```python
from build123d import *

# Parameters (mm, degrees)
SKETCH1_W                                     = 457.2
SKETCH1_H                                     = 50.8
BOSS_EXTRUDE1_DEPTH                           = 4.7625
SKETCH2_R                                     = 3.175
CUT_EXTRUDE1_DEPTH                            = 244.602
SKETCH3_R                                     = 3.175
CUT_EXTRUDE2_DEPTH                            = 244.602
SKETCH4_R                                     = 3.175
CUT_EXTRUDE3_DEPTH                            = 25.4
CSK_FOR_8_FLAT_HEAD_MACHINE_SCREW1_AT_2_COUNT = 2
CSK_FOR_8_FLAT_HEAD_MACHINE_SCREW1_AT_2_PITCH = 31.75
CSK_FOR_8_FLAT_HEAD_MACHINE_SCREW1_AT_3_COUNT = 2
CSK_FOR_8_FLAT_HEAD_MACHINE_SCREW1_AT_3_PITCH = 68.170141008
CSK_FOR_8_FLAT_HEAD_MACHINE_SCREW1_AT_4_COUNT = 2
CSK_FOR_8_FLAT_HEAD_MACHINE_SCREW1_AT_4_PITCH = 60.325
CSK_FOR_8_FLAT_HEAD_MACHINE_SCREW1_AT_5_COUNT = 2
CSK_FOR_8_FLAT_HEAD_MACHINE_SCREW1_AT_5_PITCH = 304.8
CSK_FOR_8_FLAT_HEAD_MACHINE_SCREW1_AT_6_COUNT = 2
CSK_FOR_8_FLAT_HEAD_MACHINE_SCREW1_AT_6_PITCH = 306.449184205
CSK_FOR_8_FLAT_HEAD_MACHINE_SCREW1_AT_7_COUNT = 2
CSK_FOR_8_FLAT_HEAD_MACHINE_SCREW1_AT_7_PITCH = 366.502835085
CSK_FOR_8_FLAT_HEAD_MACHINE_SCREW1_AT_8_COUNT = 2
CSK_FOR_8_FLAT_HEAD_MACHINE_SCREW1_AT_8_PITCH = 365.125


with BuildPart() as part:
    # Sketch1 → Boss-Extrude1 (new body)
    with BuildSketch(Plane(origin=(0, 0, 0), x_dir=(1, 0, 0), z_dir=(0, 1, 0))):
        with Locations((228.6, 25.4)):
            Rectangle(SKETCH1_W, SKETCH1_H)
    extrude(amount=BOSS_EXTRUDE1_DEPTH)

    # Sketch2 → Cut-Extrude1 (cut)
    with BuildSketch(Plane(origin=(0, 4.7625, 0), x_dir=(1, 0, 0), z_dir=(0, 1, 0))):
        with Locations(Location((19.05, 25.4, 0), (0, 0, 270))):
            Circle(SKETCH2_R)
        with Locations(Location((438.15, 25.4, 0), (0, 0, 270))):
            Circle(SKETCH2_R)
    extrude(amount=-CUT_EXTRUDE1_DEPTH, mode=Mode.SUBTRACT)

    # Sketch3 → Cut-Extrude2 (cut)
    with BuildSketch(Plane(origin=(0, 4.7625, 0), x_dir=(1, 0, 0), z_dir=(0, 1, 0))):
        with Locations(Location((152.4, 25.4, 0), (0, 0, 270))):
            Circle(SKETCH3_R)
        with Locations(Location((304.8, 25.4, 0), (0, 0, 270))):
            Circle(SKETCH3_R)
        with Locations(Location((228.6, 25.4, 0), (0, 0, 270))):
            Circle(SKETCH3_R)
    extrude(amount=-CUT_EXTRUDE2_DEPTH, mode=Mode.SUBTRACT)

    # Sketch4 → Cut-Extrude3 (cut)
    with BuildSketch(Plane(origin=(0, 4.7625, 0), x_dir=(1, 0, 0), z_dir=(0, 1, 0))):
        with Locations(Location((120.65, 25.4, 0), (0, 0, 270))):
            Circle(SKETCH4_R)
        with Locations(Location((336.55, 25.4, 0), (0, 0, 270))):
            Circle(SKETCH4_R)
    extrude(amount=-CUT_EXTRUDE3_DEPTH, mode=Mode.SUBTRACT)

    # Sketch5 → CSK for #8 Flat Head Machine Screw1 (revolve, cut)
    with BuildSketch(Plane(origin=(46.0375, 0, -42.06875), x_dir=(0, 0, -1), z_dir=(1, 0, 0))):
        Polygon((0, 0), (0, 4.7625), (2.15265, 4.7625), (2.15265, 2.3740728), (4.2164, 0), align=None)
    csk_for_8_flat_head_machine_screw1 = revolve(axis=Axis((46.0375, -6.35, -42.06875), (0, 1, 0)), mode=Mode.SUBTRACT)

    # CSK for #8 Flat Head Machine Screw1 at 2: CSK for #8 Flat Head Machine Screw1 ×2
    with Locations(*[(0, 0, i * CSK_FOR_8_FLAT_HEAD_MACHINE_SCREW1_AT_2_PITCH) for i in range(1, CSK_FOR_8_FLAT_HEAD_MACHINE_SCREW1_AT_2_COUNT)]):
        add(csk_for_8_flat_head_machine_screw1, mode=Mode.SUBTRACT)

    # CSK for #8 Flat Head Machine Screw1 at 3: CSK for #8 Flat Head Machine Screw1 ×2
    with Locations(*[Vector(0.8849182223819825, 0, 0.4657464328326221) * (i * CSK_FOR_8_FLAT_HEAD_MACHINE_SCREW1_AT_3_PITCH) for i in range(1, CSK_FOR_8_FLAT_HEAD_MACHINE_SCREW1_AT_3_COUNT)]):
        add(csk_for_8_flat_head_machine_screw1, mode=Mode.SUBTRACT)

    # CSK for #8 Flat Head Machine Screw1 at 4: CSK for #8 Flat Head Machine Screw1 ×2
    with Locations(*[(i * CSK_FOR_8_FLAT_HEAD_MACHINE_SCREW1_AT_4_PITCH, 0, 0) for i in range(1, CSK_FOR_8_FLAT_HEAD_MACHINE_SCREW1_AT_4_COUNT)]):
        add(csk_for_8_flat_head_machine_screw1, mode=Mode.SUBTRACT)

    # CSK for #8 Flat Head Machine Screw1 at 5: CSK for #8 Flat Head Machine Screw1 ×2
    with Locations(*[(i * CSK_FOR_8_FLAT_HEAD_MACHINE_SCREW1_AT_5_PITCH, 0, 0) for i in range(1, CSK_FOR_8_FLAT_HEAD_MACHINE_SCREW1_AT_5_COUNT)]):
        add(csk_for_8_flat_head_machine_screw1, mode=Mode.SUBTRACT)

    # CSK for #8 Flat Head Machine Screw1 at 6: CSK for #8 Flat Head Machine Screw1 ×2
    with Locations(*[Vector(0.9946184088907778, 0, 0.103606084259456) * (i * CSK_FOR_8_FLAT_HEAD_MACHINE_SCREW1_AT_6_PITCH) for i in range(1, CSK_FOR_8_FLAT_HEAD_MACHINE_SCREW1_AT_6_COUNT)]):
        add(csk_for_8_flat_head_machine_screw1, mode=Mode.SUBTRACT)

    # CSK for #8 Flat Head Machine Screw1 at 7: CSK for #8 Flat Head Machine Screw1 ×2
    with Locations(*[Vector(0.996240588195683, 0, 0.086629616364842) * (i * CSK_FOR_8_FLAT_HEAD_MACHINE_SCREW1_AT_7_PITCH) for i in range(1, CSK_FOR_8_FLAT_HEAD_MACHINE_SCREW1_AT_7_COUNT)]):
        add(csk_for_8_flat_head_machine_screw1, mode=Mode.SUBTRACT)

    # CSK for #8 Flat Head Machine Screw1 at 8: CSK for #8 Flat Head Machine Screw1 ×2
    with Locations(*[(i * CSK_FOR_8_FLAT_HEAD_MACHINE_SCREW1_AT_8_PITCH, 0, 0) for i in range(1, CSK_FOR_8_FLAT_HEAD_MACHINE_SCREW1_AT_8_COUNT)]):
        add(csk_for_8_flat_head_machine_screw1, mode=Mode.SUBTRACT)


solid = part.part
```
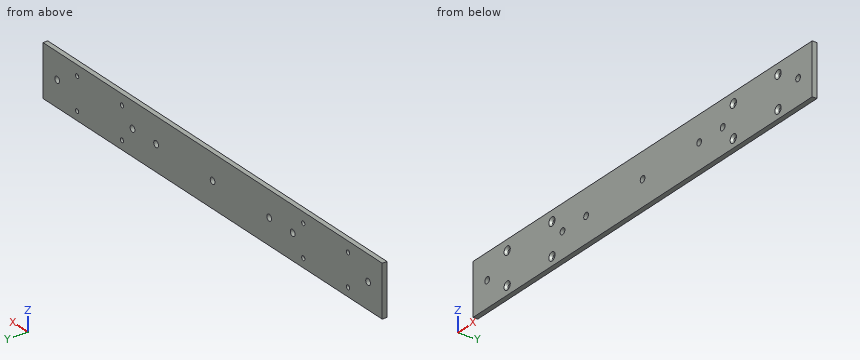
Here's how the part is built. I have some questions about the finished solid (model axes, mm). Coordinates: 2 decimals unless noted, no trailing zeros. Return JSON: item names as keys, results as strings. Group by question number.
Item 1: I need wall thicknesses on line 1 (Z direction, x = 42.5, y = 0.25); line 2 (Z direction, x = 19.5, y = 3.4); line 3 (X direction, y = 4.5, z = -43). Which ranges of each line are inside material? Lowest first, please. Write a range as from..to.
Item 2: Will these pins go through, and if not, where does the flat tip stop? P1, Ø2.5, axis at x = 106.36, z = -42.07, coming from the +Y side; P2, Ø5.5, axis at x = 46.04, z = -10.32, coming from the -Y side.
Item 3: If we section it at A-A on y = 0.75: State how many separate pieces and enclosed holes the cut face has, and give its area (3 significant figures).
Calculated:
{
 "1": {"line 1": "z = -50.8..-43.93, -40.2..-12.18, -8.45..0", "line 2": "z = -50.8..-28.54, -22.26..0", "line 3": "x = 0..44.1, 47.98..104.42, 108.3..348.9, 352.78..409.22, 413.1..457.2"},
 "2": {"P1": "passes through", "P2": "stops at y = 1.68"},
 "3": {"separate pieces": "1", "enclosed holes": "15", "area": "22,700 mm^2"}
}
